Here's how the part is built. I have some questions about the finished solid (model axes, mm). Face numbers are marked on the shaded views. A direction names the side the tool comes from. Round coordinates to 2 decimals unless told otherwise and drop trailing zeros. Write each loop counter-clockwise with the first axis right and the second up, starting at its lowest first coordinate (ties: lowest second). Pieces come first, ordered by that corner, then holes. Notation, with made-up numbers: (-29.75, 11.5) -> (-16.75, 11.5) arc R14 cw to (-16.75, 15.5) -> close; hole circle Ø10 at (13, 35). An arc over 180 degrees is marked (long way). Answer as CSV lines item,"result".
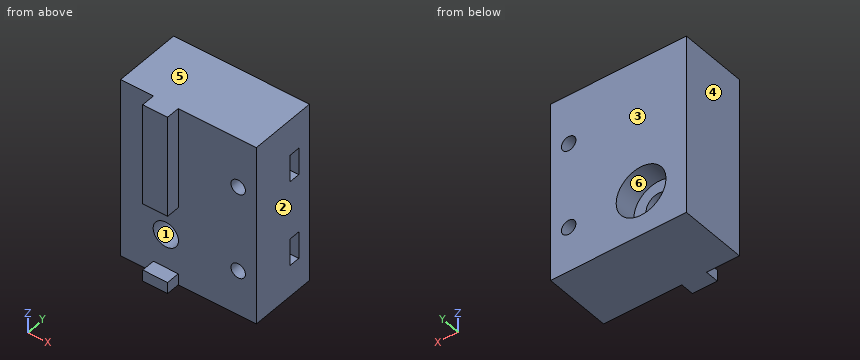
```python
from build123d import *

# Parameters (mm, degrees)
SKETCH1_W           = 30
SKETCH1_H           = 40
BOSS_EXTRUDE1_DEPTH = 15
SKETCH5_R           = 1.6
CUT_EXTRUDE3_DEPTH  = 16
SKETCH6_W           = 6
SKETCH6_H           = 2.5
CUT_EXTRUDE4_DEPTH  = 8
SKETCH10_R          = 2.8
CUT_EXTRUDE7_DEPTH  = 16
SKETCH11_R          = 5.5
CUT_EXTRUDE8_DEPTH  = 5
SKETCH12_W          = 5.5
SKETCH12_H          = 22.5
SKETCH12_H_2        = 2.5
BOSS_EXTRUDE7_DEPTH = 3


with BuildPart() as part:
    # Sketch1 → Boss-Extrude1 (new body)
    with BuildSketch(Plane(origin=(0, 0, 0), x_dir=(1, 0, 0), z_dir=(0, 1, 0))):
        with Locations((14.30324178, 20)):
            Rectangle(SKETCH1_W, SKETCH1_H)
    extrude(amount=BOSS_EXTRUDE1_DEPTH)

    # Sketch5 → Cut-Extrude3 (cut, through all)
    with BuildSketch(Plane(origin=(0, 15, 0), x_dir=(1, 0, 0), z_dir=(0, 1, 0))):
        with Locations((25.30324178, 11)):
            Circle(SKETCH5_R)
        with Locations((25.30324178, 30)):
            Circle(SKETCH5_R)
    extrude(amount=-CUT_EXTRUDE3_DEPTH, mode=Mode.SUBTRACT)

    # Sketch6 → Cut-Extrude4 (cut)
    with BuildSketch(Plane(origin=(29.30324178, 0, 0), x_dir=(0, 0, -1), z_dir=(1, 0, 0))):
        with Locations((11, 10.75)):
            Rectangle(SKETCH6_W, SKETCH6_H)
        with Locations((30, 10.75)):
            Rectangle(SKETCH6_W, SKETCH6_H)
    extrude(amount=-CUT_EXTRUDE4_DEPTH, mode=Mode.SUBTRACT)

    # Sketch10 → Cut-Extrude7 (cut, through all)
    with BuildSketch(Plane(origin=(0, 15, 0), x_dir=(1, 0, 0), z_dir=(0, 1, 0))):
        with Locations((9.30324178, 30)):
            Circle(SKETCH10_R)
    extrude(amount=-CUT_EXTRUDE7_DEPTH, mode=Mode.SUBTRACT)

    # Sketch11 → Cut-Extrude8 (cut)
    with BuildSketch(Plane(origin=(0, 15, 0), x_dir=(1, 0, 0), z_dir=(0, 1, 0))):
        with Locations((9.30324178, 30)):
            Circle(SKETCH11_R)
    extrude(amount=-CUT_EXTRUDE8_DEPTH, mode=Mode.SUBTRACT)

    # Sketch12 → Boss-Extrude7 (add)
    with BuildSketch(Plane.XZ):
        with Locations((9.30324178, -11.25)):
            Rectangle(SKETCH12_W, SKETCH12_H)
        with Locations((9.30324178, -38.75)):
            Rectangle(SKETCH12_W, SKETCH12_H_2)
    extrude(amount=BOSS_EXTRUDE7_DEPTH)


solid = part.part
```
1. For pin 1 Ø3.5 at (x, z) = (7.5, -32) entering from +Y; pin 2 Ø3.5 at (x, z) = (25.3, -11) entering from -Y; pin 3 Ø0.8 at (y, z) = (-1, -38.5) entering from +X, each with a flat end and sliding along its axis, tell me the tip position at first contact or that it passes through.
Numbers:
pin 1,"stops at y = 10"
pin 2,"stops at y = 0"
pin 3,"stops at x = 12.05"
2. If I drill on line 1 (X direction, y = 4.75, z = -30); line 2 (X direction, y = 12.3, z = -30); line 3 (Y direction, x = 26.75, z = -32), over which ranges is the centre line in solid material (lowest first)?
Numbers:
line 1,"x = -0.7 to 6.5, 12.1 to 23.7, 26.9 to 29.3"
line 2,"x = -0.7 to 3.8, 14.8 to 23.7, 26.9 to 29.3"
line 3,"y = 0 to 9.5, 12 to 15"
3. Suppose I cut it at C-C on z = -11. Please give me the cut outline in (x, y), and give its area (4 significant figures).
Numbers:
outline,"(-0.7, 0) -> (6.55, 0) -> (6.55, -3) -> (12.05, -3) -> (12.05, 0) -> (23.7, 0) -> (23.7, 9.5) -> (21.3, 9.5) -> (21.3, 12) -> (23.7, 12) -> (23.7, 15) -> (-0.7, 15) -> close; (26.9, 0) -> (29.3, 0) -> (29.3, 9.5) -> (26.9, 9.5) -> close; (26.9, 12) -> (29.3, 12) -> (29.3, 15) -> (26.9, 15) -> close"
area,"406.5 mm^2"
4. On a 3-axis mill with a long thin cutter (end or side, diameter ignored), from which of +Z, -Z, +X, -X, +Y, -Y can I reach the whole of each face in a straight line? I mean the marked faces 5 and 6. Say none if no direction works.
Numbers:
face 5,"+Z, +X, -X, +Y, -Y"
face 6,"+Y"
5. Suppose I cut it at D-D on y = 11.25. Please give me the cut outline in (x, z).
Numbers:
outline,"(-0.7, -40) -> (29.3, -40) -> (29.3, -33) -> (21.3, -33) -> (21.3, -27) -> (29.3, -27) -> (29.3, -14) -> (21.3, -14) -> (21.3, -8) -> (29.3, -8) -> (29.3, 0) -> (-0.7, 0) -> close; hole circle Ø11 at (9.3, -30)"
6. Suppose I cut it at A-A on z = -30. Please give me the cut outline in (x, y), and give its area (3 significant figures).
Numbers:
outline,"(-0.7, 0) -> (6.5, 0) -> (6.5, 10) -> (3.8, 10) -> (3.8, 15) -> (-0.7, 15) -> close; (12.1, 0) -> (23.7, 0) -> (23.7, 9.5) -> (21.3, 9.5) -> (21.3, 12) -> (23.7, 12) -> (23.7, 15) -> (14.8, 15) -> (14.8, 10) -> (12.1, 10) -> close; (26.9, 0) -> (29.3, 0) -> (29.3, 9.5) -> (26.9, 9.5) -> close; (26.9, 12) -> (29.3, 12) -> (29.3, 15) -> (26.9, 15) -> close"
area,"279 mm^2"
7. If we mould it in two halves opening along X, with no side actions, what happens to the marked faces 1, 2, 3 and 4? For each: released by +X, released by -X, zero draft, split by the parting line, or undercut.
Numbers:
face 1,"undercut"
face 2,"released by +X"
face 3,"zero draft"
face 4,"released by -X"
8. Suppose I cut it at B-B on y = 3. Please give me the cut outline in (x, z).
Numbers:
outline,"(-0.7, -40) -> (29.3, -40) -> (29.3, 0) -> (-0.7, 0) -> close; hole circle Ø5.6 at (9.3, -30); hole circle Ø3.2 at (25.3, -30); hole circle Ø3.2 at (25.3, -11)"
